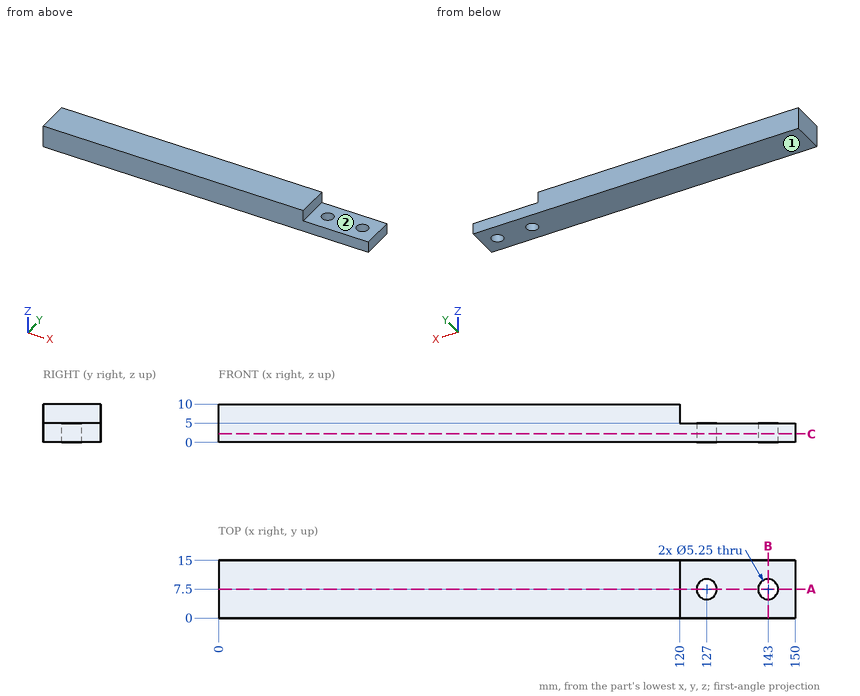
Geometry check sheet. Reference: drawing and pictorial views, mm from the part's lowest x, y, z. A direction names the side the tool comes from. Round coordinates to 2 decimals unless told otherwise and drop trailing zeros. Loops run counter-clockwise (first coordinate to the right, second up) from the corner with the lowest first, then second, coordinate; pieces in that order, holes last. Notation, with made-up numbers: (51.5, -18.75) - (83.5, -18.75) arc R14 cw to (83.5, -2.75) - close; hole circle Ø11 at (23.25, -31). An arc over 180 degrees is marked (long way). One line per question, with ' | ' between items. Start each with the question number.
1. Depth check by flat-ended pin: pin 1 (4.5 mm diameter, centred on x = 131, y = 10.5, fed in from +Z). Enter the tip coordinate at first touch or a pass-through.
2. Cross-section at C-C on z = 2.25. Record the cut outline in (x, y) (3 decimals).
3. Scan lines: line 1 (X direction, y = 7.5, z = 3.3) (3 decimals); line 2 (Y direction, x = 127, z = 1.7) (3 decimals); line 3 (X direction, y = 3, z = 7.25). Record each from-to range of solid material in increasing order. Write a range as [from, to].
4. Tool access check on the marked faces 1 and 2. Record the directions out of +Z, -Z, +X, -X, +Y, -Y that give a thin tool (end or side, any length) a straight path to the whole face; none if there is none.
5. Cross-section at B-B on x = 143. Record the cut outline in (y, z) (3 decimals), then the cut area to 4 significant figures.
6. Cross-section at A-A on y = 7.5. Record the cut outline in (x, z) (3 decimals).
Taken from the geometry:
1) pin 1: z = 5
2) outline: (0, 0) - (150, 0) - (150, 15) - (0, 15) - close; hole circle Ø5.25 at (127, 7.5); hole circle Ø5.25 at (143, 7.5)
3) line 1: [0, 124.375], [129.625, 140.375], [145.625, 150] | line 2: [0, 4.875], [10.125, 15] | line 3: [0, 120]
4) face 1: -Z, +X, -X, +Y, -Y | face 2: +Z, +X, +Y, -Y
5) outline: (0, 0) - (4.875, 0) - (4.875, 5) - (0, 5) - close; (10.125, 0) - (15, 0) - (15, 5) - (10.125, 5) - close | area: 48.75 mm²
6) outline: (0, 0) - (124.375, 0) - (124.375, 5) - (120, 5) - (120, 10) - (0, 10) - close; (129.625, 0) - (140.375, 0) - (140.375, 5) - (129.625, 5) - close; (145.625, 0) - (150, 0) - (150, 5) - (145.625, 5) - close
